Autodesk Inventor part; units mm, degrees
ref_plane "YZ Plane" through (0, 0, 0) normal (1, 0, 0) x (0, 1, 0)
ref_plane "XZ Plane" through (0, 0, 0) normal (0, 1, 0) x (-1, 0, 0)
ref_plane "XY Plane" through (0, 0, 0) normal (0, 0, 1) x (1, 0, 0)
sketch "Sketch1" plane through (0, 0, 0) normal (0, 1, 0) x (-1, 0, 0)
  line L0 (0, 0) -> (60, 0)
  line L1 (60, -81) -> (0, -81)
  line L2 (0, -81) -> (0, -40.5)
  line L3 (44.9096, -21.5055) -> (14.9096, -21.5055) construction
  line L4 (44.9096, -81) -> (44.9096, 0) construction
  line L5 (14.9096, 0) -> (14.9096, -81) construction
  circle A0 centre (39.9096, -73.5) radius 1.5
  circle A1 centre (39.9096, -7.5) radius 1.5
  circle A2 centre (19.9096, -7.5) radius 1.5
  circle A3 centre (19.9096, -73.5) radius 1.5
  line L6 (60, -40.5) -> (0, -40.5) construction
  line L7 (30, 0) -> (30, -81) construction
  circle A4 centre (30, -40.5) radius 24
  circle A5 centre (30, -40.5) radius 27.5
  circle A6 centre (57.1293, -36) radius 1.5
  circle A7 centre (57.1293, -45) radius 1.5
  circle A8 centre (25.5, -13.3707) radius 1.5
  circle A9 centre (34.5, -13.3707) radius 1.5
  circle A10 centre (2.8707, -45) radius 1.5
  circle A11 centre (2.8707, -36) radius 1.5
  circle A12 centre (34.5, -67.6293) radius 1.5
  circle A13 centre (25.5, -67.6293) radius 1.5
  arc A14 (60, -81) -> (60, 0) centre (-17.0125, -40.5) ccw
  arc A15 (-5.7831, -34.5157) -> (14.9096, -7.5073) centre (30, -40.5) ccw construction
  circle A16 centre (65.9998, -36) radius 1.5
  circle A17 centre (65.9998, -45) radius 1.5
  circle A18 centre (-5.9998, -45) radius 1.5
  circle A19 centre (-5.9998, -36) radius 1.5
  arc A20 (0, 0) -> (0, -81) centre (77.0125, -40.5) ccw
  line L8 (30, -40.5) -> (-3.3536, -73.8536) construction
  circle A21 centre (1.7157, -68.7843) radius 1.5
  circle A22 centre (11.8404, -76.1403) radius 1.5
  circle A23 centre (23.7426, -80.0075) radius 1.5
  circle A24 centre (36.2574, -80.0075) radius 1.5
  circle A25 centre (48.1596, -76.1403) radius 1.5
  circle A26 centre (58.2843, -68.7843) radius 1.5
  circle A27 centre (65.6403, -58.6596) radius 1.5
  circle A28 centre (69.5075, -46.7574) radius 1.5
  circle A29 centre (69.5075, -34.2426) radius 1.5
  circle A30 centre (65.6403, -22.3404) radius 1.5
  circle A31 centre (58.2843, -12.2157) radius 1.5
  circle A32 centre (48.1596, -4.8597) radius 1.5
  circle A33 centre (36.2574, -0.9925) radius 1.5
  circle A34 centre (23.7426, -0.9925) radius 1.5
  circle A35 centre (11.8404, -4.8597) radius 1.5
  circle A36 centre (1.7157, -12.2157) radius 1.5
  circle A37 centre (-5.6403, -22.3404) radius 1.5
  circle A38 centre (-9.5075, -34.2426) radius 1.5
  circle A39 centre (-9.5075, -46.7574) radius 1.5
  circle A40 centre (-5.6403, -58.6596) radius 1.5
  circle A41 centre (48.1596, -68.7843) radius 1.5
  circle A42 centre (48.1596, -12.2157) radius 1.5
  circle A43 centre (11.8404, -12.2157) radius 1.5
  circle A44 centre (11.8404, -68.7843) radius 1.5
  line L9 (56.4575, -33) -> (69.2906, -33)
  line L10 (37.5, -1.2094) -> (37.5, -14.0425)
  line L11 (37.5, -1.2094) -> (37.5, -14.0425)
  circle A45 centre (30, -40.5) radius 27.5
  line L12 (30, -81) -> (30, -0.5) construction
  line L13 (60, -33) -> (60, -81)
  arc A46 (60, -14.0425) -> (59.3249, -13.2961) centre (30, -40.5) ccw construction
  line L14 (55.807, -31) -> (69.4798, -31)
  circle A47 centre (48.1596, -4.8597) radius 3.25
  line L15 (51.4096, -4.8597) -> (51.4096, 0)
  line L16 (44.9096, -4.8597) -> (44.9096, 0)
  circle A48 centre (30, -40.5) radius 29.5
  line L17 (39.5, -12.5715) -> (39.5, 0)
  circle A49 centre (30, 75.5) radius 33.5
  line L18 (148.361, 0) -> (-88.361, 0)
  circle A50 centre (30, 75.5) radius 43
  arc A51 (37.7343, -1.2549) -> (13.1894, -4.2039) centre (30, -40.5) ccw
  arc A52 (-9.2451, -32.7657) -> (69.2451, -32.7657) centre (30, -40.5) ccw
  arc A53 (-9.2451, -32.7657) -> (69.2451, -32.7657) centre (30, -40.5) ccw construction
  arc A54 (37.7343, -1.2549) -> (13.1894, -4.2039) centre (30, -40.5) ccw construction
  line L19 (63.5, 75.5) -> (73, 75.5) construction
  circle A55 centre (68.25, 75.5) radius 1.5
  circle A56 centre (49.125, 108.6255) radius 1.5
  circle A57 centre (10.875, 108.6255) radius 1.5
  circle A58 centre (-8.25, 75.5) radius 1.5
  circle A59 centre (10.875, 42.3745) radius 1.5
  circle A60 centre (49.125, 42.3745) radius 1.5
  line L20 (4.193, -31) -> (-9.4798, -31)
  circle A61 centre (11.8404, -4.8597) radius 3.25
  line L21 (20.5, -12.5715) -> (20.5, 0)
  arc A62 (0, 0) -> (-12.2627, 67.5715) centre (-54.5436, 25) ccw
  arc A63 (72.2627, 67.5715) -> (60, 0) centre (114.5436, 25) ccw
  point P0 (29.9096, -21.5055)
  point P1 (30, -40.75)
  point P2 (-7.9036, 55.1945)
  point P3 (57.9285, -31)
  point P4 (2.0715, -31)
  point P5 (72.2627, 67.5715)
  point P6 (2.984, 42.0465)
  point P7 (57.016, 42.0465)
  dimension "d48" = 67
  dimension "d52" = 42
  dimension "d6" = 60
  dimension "d7" = 81
  dimension "d8" = 3
  dimension "d9" = 7.5
  dimension "d10" = 5
  dimension "d11" = 30
  dimension "d12" = 3
  dimension "d13" = 7.5
  dimension "d14" = 5
  dimension "d15" = 3
  dimension "d16" = 3
  dimension "d17" = 5
  dimension "d18" = 48
  dimension "d19" = 55
  dimension "d20" = 3
  dimension "d21" = 4.5
  dimension "d22" = 3
  dimension "d23" = 4.5
  dimension "d24" = 360
  dimension "d26" = 72.56
  dimension "d27" = 3
  dimension "d28" = 3
  dimension "d29" = 360
  dimension "d30" = 45
  dimension "d31" = 3
  dimension "d32" = 360
  dimension "d33" = 3
  dimension "d34" = 3
  dimension "d35" = 3
  dimension "d36" = 3
  dimension "d37" = 55
  dimension "d39" = 90
  dimension "d42" = 12.8331
  dimension "d43" = 12.8331
  dimension "d44" = 2
  dimension "d45" = 6.5
  dimension "d46" = 2
  dimension "d47" = 2
  dimension "d49" = 30
  dimension "d57" = 3
  dimension "d60" = 360
  dimension "d84" = 4.75
  dimension "d85" = 60
  dimension "d86" = 25
extrude "Extrusion1" add sketch "Sketch1" along normal blind 4 contours A62 A50 A63 L0 A33 A34 | L0 L21 A2 A48 L20 A20 | A62 A50 A63 | A34 L0 | L21 A2 | A14 L14 A48 L17 A1 L0 L16 A47 L15 | A33 L0 | L15 A47 L16 L0 | L17 A1 picked at (20.0279, -7.9174) picked at (39.7286, -7.0086)
ref_plane "Work Plane1" through (-30, 0, -12.5715) normal (-1, 0, 0) x (0, 0, 1)
sketch "Sketch3" plane through (-30, 0, -12.5715) normal (-1, 0, 0) x (0, 0, 1)
  line L0 (54.5715, 0) -> (84.3215, -55)
  line L1 (54.5715, 0) -> (121.5715, 0)
  line L2 (121.5715, 0) -> (54.5715, 0)
  line L3 (54.5715, 4) -> (121.5715, 4)
  line L4 (88.0715, 4) -> (88.0715, -55)
  line L5 (84.3215, -55) -> (82.0477, -55)
  line L6 (82.0477, -55) -> (52.2977, 0)
  line L7 (52.2977, 0) -> (54.5715, 0)
  line L8 (84.3215, -55) -> (84.3215, -65)
  line L9 (82.0477, -55) -> (82.0477, -65)
  line L10 (84.3215, -65) -> (82.0477, -65)
  line L11 (84.3215, -65) -> (84.3215, -75)
  line L12 (84.3215, -75) -> (82.0477, -75)
  line L13 (82.0477, -75) -> (82.0477, -65)
  point P0 (12.5715, 0)
  point P1 (88.0715, 0)
  dimension "d88" = 59
  dimension "d89" = 3.75
  dimension "d94" = 10
  dimension "d96" = 2.2738
  dimension "d98" = 10
revolve "Revolution4" add sketch "Sketch3" angle 360 about axis through (-30, 4, 75.5) along (0, -1, 0) contours L0 L5 L6 L7 | L8 L10 L9 L5
revolve "Revolution5" add sketch "Sketch3" angle 100 about axis through (-30, 4, 75.5) along (0, 1, 0) contours L11 L12 L13 L10
pattern_circular "Circular Pattern3" count 3 over 360 about axis through (-30, -60, 75.5) along (0, 1, 0) of "Revolution5"
equation "\"d11\" = 0.5 * d6"
equation "\"d12\" = d8"
equation "\"d15\" = d8"
equation "\"d16\" = d8"
equation "\"d22\" = d8"
equation "\"d27\" = d8"
equation "\"d28\" = d8"
equation "\"d31\" = d8"
equation "\"d33\" = d8"
equation "\"d34\" = d8"
equation "\"d35\" = d8"
equation "\"d36\" = d8"
properties part number "OneLensHolder"
CAD build for the part. Positions are in the model's coordinates, mm. A direction names the side the tool comes from. Round coordinates to 2 decimals unless told otherwise and drop trailing zeros. Loops run counter-clockwise (first coordinate to the right, second up) from the corner with the lowest first, then second, coordinate; pieces in that order, holes last. Notation, with made-up numbers: M 67.5,5 L 88.5,5 A28 cw 88.5,33 Z; hole C -24,-22.5 d11. An arc over 180 degrees is marked long. Return JSON: item names as keys, results as strings. Group by question number.
(1) Saw through at C-C, the plane y = -34. List the corners of the cut face in (x, z).
(2) Mould opens along Z. For faces 1 (the flat face through (-33, 0, 27)), 2 (the cylindrical face through (5.836, 1.972, -23.828)), 3 (the flat face through (4, 2, -31)) say: +Z half, -Z half, draft (parallel to the pull), parting line (faces both ways), or undercut.
(3) Wall check: probe 1 along Z at (x, y) = (-30, -60); probe 2 along X at (y, z) = (-68.5, 75.5); probe 3 along Y at (x, z) = (-7.5, 38). Give the ranges that are in metal, low to high. Write a range as [from, to].
(4) Drop flat-ended pins along their axis: P1, Ø2, axis at y = -18, z = 56, coming from the +X side; P2, Ø2.5, axis at y = -68, z = 71, coming from the +X side; P3, Ø6, axis at x = -44.5, y = -23.5, coming from the -Z side; P4, Ø2, axis at x = -26.5, z = 78.5, coming from the -Y side. Give the stop position or say it passes through.
(5) Saw through at A-A, the plane y = -46. List the corners of the cut face in (x, z).
(6) Tool access for faces 4 (the cylindrical face through (-26.335, -64.86, 80.28)), 5 (the cylindrical face through (-9.01, 1.97, -19.77)), 6 (the cylindrical face through (-11.68, 1.97, 107.36)), 7 (the cylindrical face through (-66.13, 1.97, -14.84)): list every direction of +Z, -Z, +X, -X, +Y, -Y with a clear straight run to the whole face (end or side of a thin tool).
(7) Saw through at B-B, the plane z = 27. List the corners of the cut face in (x, y).
Answer list:
{
 "1": {"outline": "C -30,75.5 d34.77; hole C -30,75.5 d30.22"},
 "2": {"face 1": "draft", "face 2": "undercut", "face 3": "-Z half"},
 "3": {"probe 1": "[69.48, 71.75], [79.25, 81.52]", "probe 2": "[-36.02, -33.75], [-26.25, -23.98]", "probe 3": "[0, 4]"},
 "4": {"P1": "x = -11.42", "P2": "x = -24.93", "P3": "z = 54.69", "P4": "y = -75"},
 "5": {"outline": "C -30,75.5 d21.78; hole C -30,75.5 d17.24"},
 "6": {"face 4": "-Y", "face 5": "-Z, +Y, -Y", "face 6": "+Y, -Y", "face 7": "-X, +Y, -Y"},
 "7": {"outline": "M -54.58,0 L -5.42,0 L -5.42,4 L -54.58,4 Z"}
}
